Verification items for this drawing (mm, ordinates from the low corner). Give positions to 0.01 mm unless a question says otherwise; leave off trailing zeros. Loops run counter-clockwise (first coordinate to the right, second up) from the corner with the lowest first, then second, coordinate; pieces in that order, holes last. Notation, with made-up numbers: M 62,-30.5 L 76,-30.5 A32 ccw 76,3.5 Z; hole C -24.75,-35.5 d7. An arc over 180 degrees is marked long. Use a Markdown table: item, result.
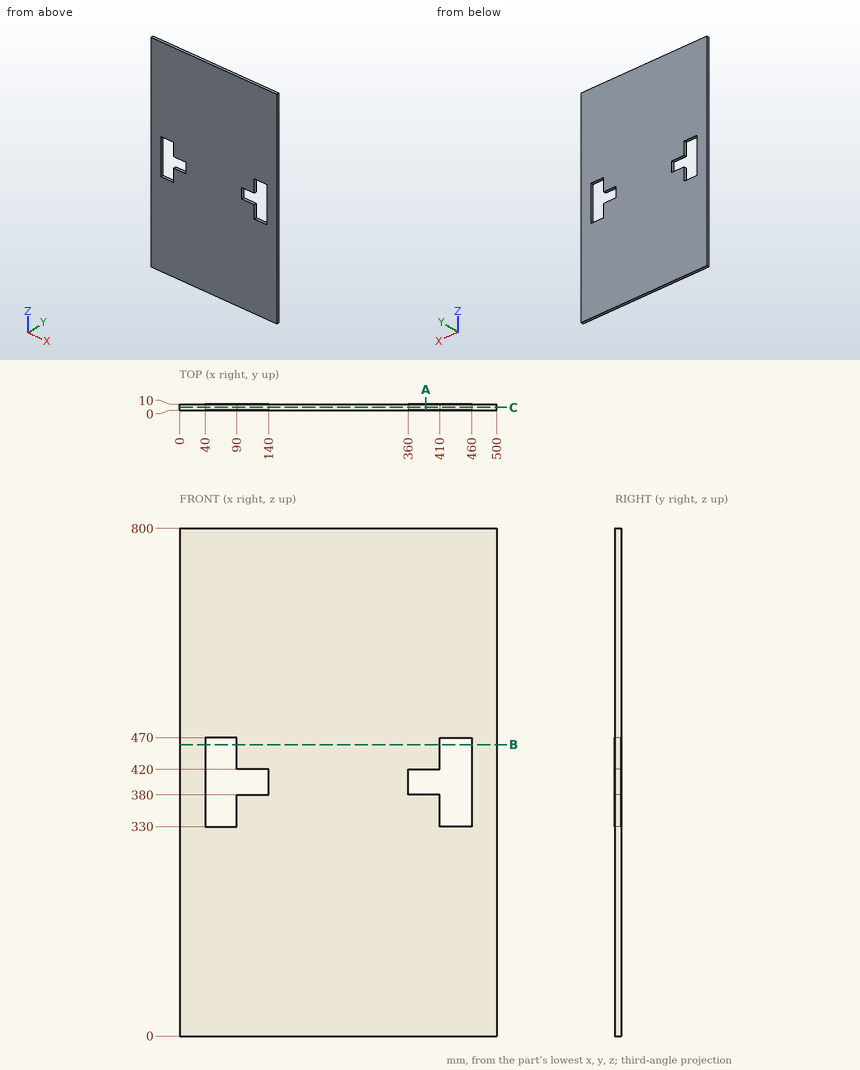
(1) Cross-section at A-A on x = 388. Record the cut outline in (y, z).
Results below:
| item | result |
|---|---|
| outline | M 0,0 L 10,0 L 10,380 L 0,380 Z; M 0,420 L 10,420 L 10,800 L 0,800 Z |
(2) Cross-section at C-C on y = 4.75. Record the cut outline in (x, z), then the cut area to 3 significant figures.
Results below:
| item | result |
|---|---|
| outline | M 0,0 L 500,0 L 500,800 L 0,800 Z; hole M 40,330 L 90,330 L 90,380 L 140,380 L 140,420 L 90,420 L 90,470 L 40,470 Z; hole M 360,380 L 410,380 L 410,330 L 460,330 L 460,470 L 410,470 L 410,420 L 360,420 Z |
| area | 382,000 mm^2 |
(3) Material ranges on line 1 (X direction, y = 5.25, z = 373.5); line 2 (Z direction, x = 116.5, y = 6); line 3 (Z direction, x = 45, y = 5), recorded low to high.
Results below:
| item | result |
|---|---|
| line 1 | 0 to 40, 90 to 410, 460 to 500 |
| line 2 | 0 to 380, 420 to 800 |
| line 3 | 0 to 330, 470 to 800 |
(4) Cross-section at B-B on z = 459. Record the cut outline in (x, y).
Results below:
| item | result |
|---|---|
| outline | M 0,0 L 40,0 L 40,10 L 0,10 Z; M 90,0 L 410,0 L 410,10 L 90,10 Z; M 460,0 L 500,0 L 500,10 L 460,10 Z |
